Check sheet for the modelled part. Datum: model origin and axes. Units: mm. Give positions to 0.01 mm unless a question says otherwise; leave off trailing zeros. Order: outer loops, then holes, each group sorted by start corner. A loop starts at its lowest first (then second) coordinate and runs counter-clockwise, first axis right, second up. Notation, with made-up numbers: (68.5, 0) -> (80.5, 0) arc R20 cw to (80.5, 10) -> close; hole circle Ø4 at (48.5, 64). An arc over 180 degrees is marked (long way). One line per question, with ' | ' between items.
```python
from build123d import *

# Parameters (mm, degrees)
SKETCH1_R           = 6.15
BOSS_EXTRUDE1_DEPTH = 17
BOSS_EXTRUDE2_START = -73.4
SKETCH1_2_R         = 6.15
BOSS_EXTRUDE2_DEPTH = 73.4
SKETCH4_W           = 9.7
SKETCH4_H           = 9.7
CUT_EXTRUDE1_DEPTH  = 1.5
FILLET1_R           = 1


with BuildPart() as part:
    # Sketch1 → Boss-Extrude1 (new body)
    with BuildSketch(Plane.XY):
        with Locations((-46.956139987, 36.685790659)):
            Circle(SKETCH1_R)
    extrude(amount=BOSS_EXTRUDE1_DEPTH)

    # Sketch1<2> → Boss-Extrude2 (add)
    with BuildSketch(Plane.XY.offset(BOSS_EXTRUDE2_START)):
        with Locations((-46.956139987, 36.685790659)):
            Circle(SKETCH1_2_R)
    extrude(amount=BOSS_EXTRUDE2_DEPTH)

    # Sketch3 → Loft1 section 0
    with BuildSketch(Plane(origin=(0, 0, -121.9), x_dir=(-1, 0, 0), z_dir=(0, 0, -1))):
        with BuildLine():
            Line((41.256139987, 42.385790659), (52.656139987, 42.385790659))
            Line((52.656139987, 42.385790659), (52.656139987, 30.985790659))
            Line((52.656139987, 30.985790659), (41.256139987, 30.985790659))
            Line((41.256139987, 30.985790659), (41.256139987, 42.385790659))
        make_face()
    # Sketch2 for Loft1 → Loft1 section 1
    with BuildSketch(Plane(origin=(0, 0, -73.4), x_dir=(-1, 0, 0), z_dir=(0, 0, -1))):
        with BuildLine():
            # circular arc as an exact rational Bezier (weights 1, cos(half-angle), 1)
            Bezier((42.006392519, 41.635538128), (46.956139988, 46.585285594), (51.905887456, 41.635538128), weights=[1, 0.707106781, 1])
            Bezier((51.905887456, 41.635538128), (56.855634922, 36.68579066), (51.905887456, 31.736043191), weights=[1, 0.707106781, 1])
            Bezier((51.905887456, 31.736043191), (46.956139987, 26.786295722), (42.006392519, 31.736043191), weights=[1, 0.707106781, 1])
            Bezier((42.006392519, 31.736043191), (37.05664505, 36.685790659), (42.006392519, 41.635538128), weights=[1, 0.707106781, 1])
        make_face()
    loft()

    # Sketch4 → Cut-Extrude1 (cut)
    with BuildSketch(Plane(origin=(0, 0, -121.9), x_dir=(-1, 0, 0), z_dir=(0, 0, -1))):
        with Locations((46.956139987, 36.685790659)):
            Rectangle(SKETCH4_W, SKETCH4_H)
    extrude(amount=-CUT_EXTRUDE1_DEPTH, mode=Mode.SUBTRACT)

    # Fillet1
    fillet1_edges = [part.edges().sort_by_distance(p)[0] for p in [
        (-51.806139987, 41.535790659, -121.15),
        (-51.806139987, 31.835790659, -121.15),
        (-42.106139987, 31.835790659, -121.15),
        (-42.106139987, 41.535790659, -121.15),
    ]]
    fillet(fillet1_edges, radius=FILLET1_R)


solid = part.part
```
Q1. Mould release check, pull along Y, two halves, no side actions. Record for faces 1 (the face through (-41.09, 38.53, -28.83)), 2 (the face through (-47, 37, -120.4)), 3 (the face through (-47, 30, -73.4)): pulls with the +Y half, pulls with the -Y half, needs draft (parallel to the pull), parting line crosses it, or undercut.
Result sheet:
face 1: parting line crosses it | face 2: undercut | face 3: needs draft
Q2. Thickness scan on line 1 (Z direction, x = -42.75, y = 37.5); line 2 (Y direction, x = -51.25, z = -99); line 3 (X direction, y = 37, z = -44). Record the ranges inside material, lowest first.
Result sheet:
line 1: z = -120.4 to 17 | line 2: y = 31 to 42.37 | line 3: x = -53.1 to -40.81
Q3. Section check A-A (z = -35.5). Enter the section's corners in (x, y), and give its area (3 significant figures).
Result sheet:
outline: circle Ø12.3 at (-46.96, 36.69) | area: 119 mm2
Q4. Depth check by flat-ended pin: pin 1 Ø0.8 at (y, z) = (36.5, -121) entering from -X; pin 2 Ø1 at (y, z) = (32, -49.5) entering from -X; pin 3 Ø8 at (x, y) = (-43.5, 39) entering from -Z; pin 4 Ø2 at (y, z) = (31.5, -29.5) entering from +X. Enter the tip coordinate at first touch or a pass-through.
Result sheet:
pin 1: stops at x = -52.69 | pin 2: stops at x = -51.46 | pin 3: stops at z = -121.9 | pin 4: stops at x = -42.45
